Verification items for the finished model (mm, model axes). A direction names the side the tool comes from. Round coordinates to 2 decimals unless told otherwise and drop trailing zeros. Write each loop counter-clockwise with the first axis right and the second up, starting at its lowest first coordinate (ties: lowest second). Pieces come first, ordered by that corner, then holes. Notation, with made-up numbers: M -21,-25.5 L 21,-25.5 A21 ccw 21,-5.5 Z; hole C 32,-7.5 d3. An arc over 180 degrees is marked long. Answer in a Markdown table with one row per item. Add a question column.
1. Sectioned sample at B-B on x = -30. Record the cut outline in (y, z).
2. Go/stop test with a flat-tipped pin: pin 1 Ø13 at (x, z) = (-5, -1) entering from +Y. Record where the tip stops, or that it passes through.
3. Sectioned sample at A-A on z = 30. Record the cut outline in (x, y).
4. Sectioned sample at C-C on y = 6.5. Record the cut outline in (x, z), plus the area to 3 significant figures.
5. Set-up check for faces 4 (the cylindrical face through (-36.93, 0.11, 36.9)), 5 (the flat face through (31, 2.5, -28)): record each of +Z, -Z, +X, -X, +Y, -Y from which the full face is reachable in a straight line by a thin tool's end or side.
6. Sectioned sample at D-D on x = 0. Record the cut outline in (y, z), plus the area to 3 significant figures.
7. Draft check along X on faces 1 (the cylindrical face through (36.9, 0.11, -36.93)), 2 (the flat face through (0, 0, -37.5)), 3 (the cylindrical face through (-10.316, 5.035, 7.91)). Enter one of: pulls with the +X half, pulls with the -X half, needs draft (parallel to the pull), parting line crosses it, or undercut.
8. Material ranges on probe 1 along X at (y, z) = (4.75, -30); probe 2 along Z at (x, y) = (-30, 0), recorded low to high.
```python
from build123d import *

# Parameters (mm, degrees)
SKETCH1_W           = 75
SKETCH1_H           = 15
BOSS_EXTRUDE1_DEPTH = 37.5
SKETCH2_R           = 13
SKETCH2_R_2         = 3
CUT_EXTRUDE1_DEPTH  = 5
SKETCH3_R           = 2
CUT_EXTRUDE2_DEPTH  = 11
FILLET1_R           = 2


with BuildPart() as part:
    # Sketch1 → Boss-Extrude1 (new body, symmetric)
    with BuildSketch(Plane.XY):
        Rectangle(SKETCH1_W, SKETCH1_H)
    extrude(amount=BOSS_EXTRUDE1_DEPTH, both=True)

    # Sketch2 → Cut-Extrude1 (cut)
    with BuildSketch(Plane(origin=(0, 7.5, 0), x_dir=(1, 0, 0), z_dir=(0, 1, 0))):
        Circle(SKETCH2_R)
        with Locations((-30, 30)):
            Circle(SKETCH2_R_2)
        with Locations((-30, -30)):
            Circle(SKETCH2_R_2)
        with Locations((30, -30)):
            Circle(SKETCH2_R_2)
        with Locations((30, 30)):
            Circle(SKETCH2_R_2)
    extrude(amount=-CUT_EXTRUDE1_DEPTH, mode=Mode.SUBTRACT)

    # Sketch3 → Cut-Extrude2 (cut, through all)
    with BuildSketch(Plane(origin=(0, 2.5, 0), x_dir=(1, 0, 0), z_dir=(0, 1, 0))):
        with Locations((-30, 30)):
            Circle(SKETCH3_R)
        with Locations((30, 30)):
            Circle(SKETCH3_R)
        with Locations((30, -30)):
            Circle(SKETCH3_R)
        with Locations((-30, -30)):
            Circle(SKETCH3_R)
    extrude(amount=-CUT_EXTRUDE2_DEPTH, mode=Mode.SUBTRACT)

    # Fillet1
    fillet1_edges = [part.edges().sort_by_distance(p)[0] for p in [
        (-37.5, 0, 37.5),
        (37.5, 0, 37.5),
        (-37.5, 0, -37.5),
        (37.5, 0, -37.5),
    ]]
    fillet(fillet1_edges, radius=FILLET1_R)


solid = part.part
```
Geometry check:
| question | item | result |
|---|---|---|
| 1 | outline | M -7.5,-37.5 L 7.5,-37.5 L 7.5,-33 L 2.5,-33 L 2.5,-32 L -7.5,-32 Z; M -7.5,-28 L 2.5,-28 L 2.5,-27 L 7.5,-27 L 7.5,27 L 2.5,27 L 2.5,28 L -7.5,28 Z; M -7.5,32 L 2.5,32 L 2.5,33 L 7.5,33 L 7.5,37.5 L -7.5,37.5 Z |
| 2 | pin 1 | stops at y = 2.5 |
| 3 | outline | M -37.5,-7.5 L -32,-7.5 L -32,2.5 L -33,2.5 L -33,7.5 L -37.5,7.5 Z; M -28,-7.5 L 28,-7.5 L 28,2.5 L 27,2.5 L 27,7.5 L -27,7.5 L -27,2.5 L -28,2.5 Z; M 32,-7.5 L 37.5,-7.5 L 37.5,7.5 L 33,7.5 L 33,2.5 L 32,2.5 Z |
| 4 | outline | M -37.5,-35.5 A2 ccw -35.5,-37.5 L 35.5,-37.5 A2 ccw 37.5,-35.5 L 37.5,35.5 A2 ccw 35.5,37.5 L -35.5,37.5 A2 ccw -37.5,35.5 Z; hole C -30,-30 d6; hole C -30,30 d6; hole C 0,0 d26; hole C 30,-30 d6; hole C 30,30 d6 |
| 4 | area | 4,980 mm2 |
| 5 | face 4 | +Z, -X, +Y, -Y |
| 5 | face 5 | +Y |
| 6 | outline | M -7.5,-37.5 L 7.5,-37.5 L 7.5,-13 L 2.5,-13 L 2.5,13 L 7.5,13 L 7.5,37.5 L -7.5,37.5 Z |
| 6 | area | 995 mm2 |
| 7 | face 1 | pulls with the +X half |
| 7 | face 2 | needs draft |
| 7 | face 3 | undercut |
| 8 | probe 1 | x = -37.5 to -33, -27 to 27, 33 to 37.5 |
| 8 | probe 2 | z = -37.5 to -32, -28 to 28, 32 to 37.5 |
